Verification items for this drawing (mm, ordinates from the low corner). A direction names the side the tool comes from. Give positions to 0.01 mm unless a question says otherwise; leave off trailing zeros. Loops run counter-clockwise (first coordinate to the right, second up) from the corner with the lowest first, then second, coordinate; pieces in that order, holes last. Notation, with made-up numbers: (-13, 9) -> (21, 9) arc R19 cw to (21, 31) -> close; hole circle Ø11 at (57, 60.5). An arc over 180 degrees is marked (long way). Answer as a JSON object with one key per item and string values.
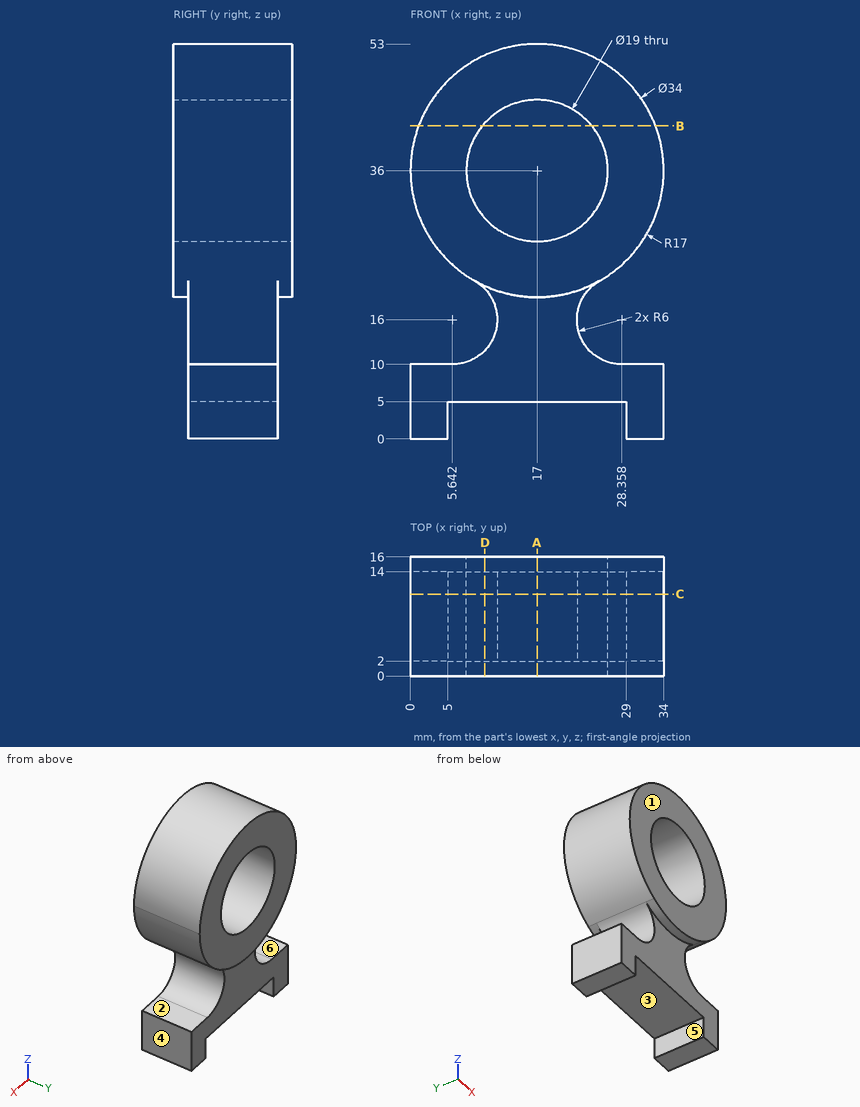
1) Section check B-B on z = 42. Record the cut outline in (x, y), plus the area to 3 significant figures.
Geometry check:
{"outline": "(1.09, 0) -> (9.63, 0) -> (9.63, 16) -> (1.09, 16) -> close; (24.37, 0) -> (32.91, 0) -> (32.91, 16) -> (24.37, 16) -> close", "area": "273 mm2"}
2) Section check A-A on x = 17. Record the cut outline in (y, z), plus the area to 3 significant figures.
Geometry check:
{"outline": "(0, 19) -> (2, 19) -> (2, 5) -> (14, 5) -> (14, 19) -> (16, 19) -> (16, 26.5) -> (0, 26.5) -> close; (0, 45.5) -> (16, 45.5) -> (16, 53) -> (0, 53) -> close", "area": "408 mm2"}
3) Section check D-D on x = 10. Record the cut outline in (y, z).
Geometry check:
{"outline": "(0, 20.51) -> (2, 20.51) -> (2, 20.12) -> (14, 20.12) -> (14, 20.51) -> (16, 20.51) -> (16, 29.58) -> (0, 29.58) -> close; (0, 42.42) -> (16, 42.42) -> (16, 51.49) -> (0, 51.49) -> close; (2, 5) -> (14, 5) -> (14, 11.88) -> (2, 11.88) -> close"}
4) Depth check by flat-ended pin: P1, Ø2, axis at x = 17, y = 5.5, coming from the -Z side; P2, Ø6, axis at x = 22, y = 6, coming from the +Z side; P3, Ø4.5, axis at x = 2.5, y = 9, coming from the +Z side; P4, Ø17, axis at x = 17, z = 11, coming from the -Y side. Enter the tip coordinate at first touch or a pass-through.
Geometry check:
{"P1": "stops at z = 5", "P2": "stops at z = 52.88", "P3": "stops at z = 47.79", "P4": "stops at y = 0"}
5) Section check C-C on y = 11. Record the cut outline in (x, z) (1 decimal), plus the area to 3 significant figures.
Geometry check:
{"outline": "(0, 0) -> (5, 0) -> (5, 5) -> (29, 5) -> (29, 0) -> (34, 0) -> (34, 10) -> (28.4, 10) arc R6 cw to (25.4, 21.2) arc R17 ccw (long way) to (8.6, 21.2) arc R6 cw to (5.6, 10) -> (0, 10) -> close; hole circle Ø19 at (17, 36)", "area": "964 mm2"}
6) Tool access check on the marked faces 4, 5 and 6. Record the directions out of +Z, -Z, +X, -X, +Y, -Y that give a thin tool (end or side, any length) a straight path to the whole face; none if there is none.
Geometry check:
{"face 4": "+Z, -Z, +X, +Y, -Y", "face 5": "-Z, +Y, -Y", "face 6": "-X, +Y, -Y"}
7) Draft check along Z on the marked faces 1, 2 and 3. Enter one of: pulls with the +Z half, pulls with the -Z half, needs draft (parallel to the pull), parting line crosses it, or undercut.
Geometry check:
{"face 1": "needs draft", "face 2": "undercut", "face 3": "pulls with the -Z half"}
8) Material ranges on line 1 along Z through (x, y) = (17, 9.5); line 2 along Z through (x, y) = (21, 3); line 3 along X through (y, z) = (10, 30.5) (1 decimal), recorded low to high. Write a range as from..to.
Geometry check:
{"line 1": "z = 5..26.5, 45.5..53", "line 2": "z = 5..27.38, 44.62..52.52", "line 3": "x = 0.9..9.3, 24.7..33.1"}
